Source: CAD feature listing. Evaluate the final solid. Frame: model axes, mm. Face numbers are marked on the shaded views. A direction names the side the tool comes from. Round coordinates to 2 decimals unless told otherwise and drop trailing zeros. Write each loop counter-clockwise with the first axis right and the second up, starting at its lowest first coordinate (ties: lowest second). Pieces come first, ordered by that corner, then holes.
from build123d import *

# Parameters (mm, degrees)
SKETCH1_R           = 3.5014085
SKETCH1_R_2         = 2.1
BOSS_EXTRUDE3_DEPTH = 2


with BuildPart() as part:
    # Sketch1 → Boss-Extrude3 (new body)
    # profile 1 of 12: a face of its own
    with BuildSketch(Plane(origin=(0, 0, 0), x_dir=(1, 0, 0), z_dir=(0, 1, 0))):
        with BuildLine():
            ThreePointArc((-3.5014085, 0), (-3.359576854, 0.986460769), (-2.945572271, 1.893004354))
            ThreePointArc((-2.945572271, 1.893004354), (-3.033257635, 1.810305959), (-3.149447141, 1.778247481))
            Line((-3.149447141, 1.778247481), (-4.615566287, 1.740476447))
            ThreePointArc((-4.615566287, 1.740476447), (-4.978126808, 1.461709916), (-4.823834054, 1.03118157))
            Line((-4.823834054, 1.03118157), (-3.610876706, 0.206762702))
            ThreePointArc((-3.610876706, 0.206762702), (-3.530463995, 0.116976603), (-3.5014085, 0))
        make_face()
    # profile 2 of 12: a face of its own
    with BuildSketch(Plane(origin=(0, 0, 0), x_dir=(1, 0, 0), z_dir=(0, 1, 0))):
        with BuildLine():
            ThreePointArc((-2.945572271, 1.893004354), (-2.29293494, 2.646187984), (-1.454537658, 3.1849932))
            ThreePointArc((-1.454537658, 3.1849932), (-1.573013407, 3.162829171), (-1.688090363, 3.198676652))
            Line((-1.688090363, 3.198676652), (-2.941888835, 3.95954549))
            ThreePointArc((-2.941888835, 3.95954549), (-3.39760672, 3.921047178), (-3.500568593, 3.475446725))
            Line((-3.500568593, 3.475446725), (-2.925878429, 2.126127187))
            ThreePointArc((-2.925878429, 2.126127187), (-2.906772982, 2.007119921), (-2.945572271, 1.893004354))
        make_face()
    # profile 3 of 12: a face of its own
    with BuildSketch(Plane(origin=(0, 0, 0), x_dir=(1, 0, 0), z_dir=(0, 1, 0))):
        with BuildLine():
            ThreePointArc((-1.454537658, 3.1849932), (-0.498302384, 3.46576921), (0.498302384, 3.46576921))
            ThreePointArc((0.498302384, 3.46576921), (0.386651462, 3.511176468), (0.309223179, 3.603548588))
            Line((0.309223179, 3.603548588), (-0.334182465, 4.921486817))
            ThreePointArc((-0.334182465, 4.921486817), (-0.738370505, 5.135479665), (-1.065897337, 4.816282101))
            Line((-1.065897337, 4.816282101), (-1.311934425, 3.370461313))
            ThreePointArc((-1.311934425, 3.370461313), (-1.360202085, 3.260016845), (-1.454537658, 3.1849932))
        make_face()
    # profile 4 of 12: a face of its own
    with BuildSketch(Plane(origin=(0, 0, 0), x_dir=(1, 0, 0), z_dir=(0, 1, 0))):
        with BuildLine():
            ThreePointArc((0.498302384, 3.46576921), (1.454537658, 3.1849932), (2.29293494, 2.646187984))
            ThreePointArc((2.29293494, 2.646187984), (2.223557225, 2.744750046), (2.208360546, 2.864319308))
            Line((2.208360546, 2.864319308), (2.379624476, 4.320890853))
            ThreePointArc((2.379624476, 4.320890853), (2.155293128, 4.719433645), (1.707188792, 4.62798194))
            Line((1.707188792, 4.62798194), (0.71853949, 3.544697787))
            ThreePointArc((0.71853949, 3.544697787), (0.618223363, 3.477881456), (0.498302384, 3.46576921))
        make_face()
    # profile 5 of 12: a face of its own
    with BuildSketch(Plane(origin=(0, 0, 0), x_dir=(1, 0, 0), z_dir=(0, 1, 0))):
        with BuildLine():
            ThreePointArc((2.29293494, 2.646187984), (2.945572271, 1.893004354), (3.359576854, 0.986460769))
            ThreePointArc((3.359576854, 0.986460769), (3.354499279, 1.106884877), (3.406359043, 1.215688886))
            Line((3.406359043, 1.215688886), (4.33791746, 2.348442573))
            ThreePointArc((4.33791746, 2.348442573), (4.364666422, 2.805000788), (3.938254542, 2.970330213))
            Line((3.938254542, 2.970330213), (2.520882193, 2.593517759))
            ThreePointArc((2.520882193, 2.593517759), (2.400367261, 2.591543277), (2.29293494, 2.646187984))
        make_face()
    # profile 6 of 12: a face of its own
    with BuildSketch(Plane(origin=(0, 0, 0), x_dir=(1, 0, 0), z_dir=(0, 1, 0))):
        with BuildLine():
            Line((4.918952301, 0.369619631), (3.522862612, 0.818914167))
            ThreePointArc((3.522862612, 0.818914167), (3.420411514, 0.882408419), (3.359576854, 0.986460769))
            ThreePointArc((3.359576854, 0.986460769), (3.46576921, 0.498302384), (3.5014085, 0))
            ThreePointArc((3.5014085, 0), (3.46576921, -0.498302384), (3.359576854, -0.986460769))
            ThreePointArc((3.359576854, -0.986460769), (3.420411514, -0.882408419), (3.522862612, -0.818914167))
            Line((3.522862612, -0.818914167), (4.918952301, -0.369619631))
            ThreePointArc((4.918952301, -0.369619631), (5.188288966, 0), (4.918952301, 0.369619631))
        make_face()
    # profile 7 of 12: a face of its own
    with BuildSketch(Plane(origin=(0, 0, 0), x_dir=(1, 0, 0), z_dir=(0, 1, 0))):
        with BuildLine():
            ThreePointArc((3.406359043, -1.215688886), (3.354499279, -1.106884877), (3.359576854, -0.986460769))
            ThreePointArc((3.359576854, -0.986460769), (2.945572271, -1.893004354), (2.29293494, -2.646187984))
            ThreePointArc((2.29293494, -2.646187984), (2.400367261, -2.591543277), (2.520882193, -2.593517759))
            Line((2.520882193, -2.593517759), (3.938254542, -2.970330213))
            ThreePointArc((3.938254542, -2.970330213), (4.364666422, -2.805000788), (4.33791746, -2.348442573))
            Line((4.33791746, -2.348442573), (3.406359043, -1.215688886))
        make_face()
    # profile 8 of 12: a face of its own
    with BuildSketch(Plane(origin=(0, 0, 0), x_dir=(1, 0, 0), z_dir=(0, 1, 0))):
        with BuildLine():
            ThreePointArc((2.208360546, -2.864319308), (2.223557225, -2.744750046), (2.29293494, -2.646187984))
            ThreePointArc((2.29293494, -2.646187984), (1.454537658, -3.1849932), (0.498302384, -3.46576921))
            ThreePointArc((0.498302384, -3.46576921), (0.618223363, -3.477881456), (0.71853949, -3.544697787))
            Line((0.71853949, -3.544697787), (1.707188792, -4.62798194))
            ThreePointArc((1.707188792, -4.62798194), (2.155293128, -4.719433645), (2.379624476, -4.320890853))
            Line((2.379624476, -4.320890853), (2.208360546, -2.864319308))
        make_face()
    # profile 9 of 12: a face of its own
    with BuildSketch(Plane(origin=(0, 0, 0), x_dir=(1, 0, 0), z_dir=(0, 1, 0))):
        with BuildLine():
            ThreePointArc((0.309223179, -3.603548588), (0.386651462, -3.511176468), (0.498302384, -3.46576921))
            ThreePointArc((0.498302384, -3.46576921), (-0.498302384, -3.46576921), (-1.454537658, -3.1849932))
            ThreePointArc((-1.454537658, -3.1849932), (-1.360202085, -3.260016845), (-1.311934425, -3.370461313))
            Line((-1.311934425, -3.370461313), (-1.065897337, -4.816282101))
            ThreePointArc((-1.065897337, -4.816282101), (-0.738370505, -5.135479665), (-0.334182465, -4.921486817))
            Line((-0.334182465, -4.921486817), (0.309223179, -3.603548588))
        make_face()
    # profile 10 of 12: a face of its own
    with BuildSketch(Plane(origin=(0, 0, 0), x_dir=(1, 0, 0), z_dir=(0, 1, 0))):
        with BuildLine():
            ThreePointArc((-1.688090363, -3.198676652), (-1.573013407, -3.162829171), (-1.454537658, -3.1849932))
            ThreePointArc((-1.454537658, -3.1849932), (-2.29293494, -2.646187984), (-2.945572271, -1.893004354))
            ThreePointArc((-2.945572271, -1.893004354), (-2.906772982, -2.007119921), (-2.925878429, -2.126127187))
            Line((-2.925878429, -2.126127187), (-3.500568593, -3.475446725))
            ThreePointArc((-3.500568593, -3.475446725), (-3.39760672, -3.921047178), (-2.941888835, -3.95954549))
            Line((-2.941888835, -3.95954549), (-1.688090363, -3.198676652))
        make_face()
    # profile 11 of 12: a face of its own
    with BuildSketch(Plane(origin=(0, 0, 0), x_dir=(1, 0, 0), z_dir=(0, 1, 0))):
        with BuildLine():
            ThreePointArc((-2.945572271, -1.893004354), (-3.359576854, -0.986460769), (-3.5014085, 0))
            ThreePointArc((-3.5014085, 0), (-3.530463995, -0.116976603), (-3.610876706, -0.206762702))
            Line((-3.610876706, -0.206762702), (-4.823834054, -1.03118157))
            ThreePointArc((-4.823834054, -1.03118157), (-4.978126808, -1.461709916), (-4.615566287, -1.740476447))
            Line((-4.615566287, -1.740476447), (-3.149447141, -1.778247481))
            ThreePointArc((-3.149447141, -1.778247481), (-3.033257635, -1.810305959), (-2.945572271, -1.893004354))
        make_face()
    # profile 12 of 12: a face of its own
    with BuildSketch(Plane(origin=(0, 0, 0), x_dir=(1, 0, 0), z_dir=(0, 1, 0))):
        Circle(SKETCH1_R)
        with Locations(Location((0, 0, 0), (0, 0, 270))):
            Circle(SKETCH1_R_2, mode=Mode.SUBTRACT)
    extrude(amount=BOSS_EXTRUDE3_DEPTH)


solid = part.part
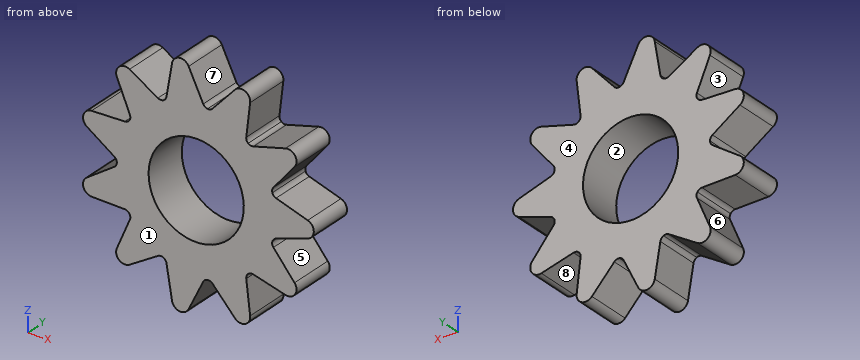
1) Section query C-C on z = -3.75. Return the cut outline in (x, y).
Taken from the geometry:
outline: (-3.51, 0) - (-2.6, 0) - (-2.6, 2) - (-3.51, 2) - close; (-1.25, 0) - (0.24, 0) - (0.24, 2) - (-1.25, 2) - close; (0.91, 0) - (2.31, 0) - (2.31, 2) - (0.91, 2) - close
2) Material intervals for line 1 (X direction, y = 1.3, z = 0); line 2 (X direction, y = 1.85, z = 4.25); line 3 (Z direction, x = -4.5, y = 0.85), sorted ascending.
Taken from the geometry:
line 1: x = -3.5 to -2.1, 2.1 to 5.19
line 2: x = -1.16 to -0.01, 1.36 to 2.37
line 3: z = -1.74 to -0.81, 0.81 to 1.74
3) Pull-direction query (X, two-part tool) for the marked faces 1, 2 and 3; classes: released by +X, released by -X, zero draft, split by the parting line, or undercut.
Taken from the geometry:
face 1: zero draft
face 2: undercut
face 3: released by -X
4) Section query B-B on x = 0. Return the cut outline in (y, z).
Taken from the geometry:
outline: (0, -4.24) - (2, -4.24) - (2, -2.1) - (0, -2.1) - close; (0, 2.1) - (2, 2.1) - (2, 4.24) - (0, 4.24) - close
5) Section query A-A on z = -1.5. Return the cut outline in (x, y).
Taken from the geometry:
outline: (-4.96, 0) - (-1.47, 0) - (-1.47, 2) - (-4.96, 2) - close; (1.47, 0) - (3.64, 0) - (3.64, 2) - (1.47, 2) - close
6) Reachability of the marked faces 4, 5, 6, 7 and 8 from +Z, -Z, +X, -X, +Y, -Y: full face, straight path, thin tool, end or side. Return the list, or none.
Taken from the geometry:
face 4: +Z, -Z, +X, -X, +Y
face 5: +X, +Y, -Y
face 6: -X, +Y, -Y
face 7: +Z, +Y, -Y
face 8: -Z, +Y, -Y
7) Section query D-D on x = 2.75. Return the cut outline in (y, z).
Taken from the geometry:
outline: (0, -2.65) - (2, -2.65) - (2, 2.65) - (0, 2.65) - close
